from build123d import *

# Parameters (mm, degrees)
CUT_EXTRUDE1_DEPTH       = 12.7
SKETCH10_W               = 4.827435186
SKETCH10_H               = 6.985
FILLET1_R                = 5.08
CIRPATTERN1_COUNT        = 6
FILLET1_OF_CIRPATTERN1_R = 5.08
FILLET2_R                = 0.762
FILLET3_R                = 0.508


with BuildPart() as part:
    # Sketch1 → Revolve1 (revolve)
    with BuildSketch(Plane.XY, mode=Mode.PRIVATE) as revolve1_sk:
        Polygon((71.12, 36.5125), (71.12, 15.5575), (75.565, 15.5575), (75.565, 6.0325), (64.77, 6.0325), (64.77, 18.7325), (67.818, 18.7325), (67.818, 21.9075), (64.77, 21.9075), (64.77, 36.5125), align=None)
    revolve(revolve1_sk.sketch.rotate(Axis((0, 60.757954545, 0), (0, -1, 0)), 180), axis=Axis((0, 60.757954545, 0), (0, -1, 0)))

    # Sketch2 → Cut-Extrude1 (cut)
    with BuildSketch(Plane(origin=(0, 36.5125, 0), x_dir=(1, 0, 0), z_dir=(0, 1, 0))):
        with BuildLine():
            Line((-8.659215821, -70.590880299), (-8.659215821, -65.726040634))
            ThreePointArc((-8.659215821, -65.726040634), (-5.173944735, -66.0917902), (-1.674215821, -66.272855962))
            Line((-1.674215821, -66.272855962), (-1.674215821, -71.100291148))
            ThreePointArc((-1.674215821, -71.100291148), (-5.172990163, -70.931618992), (-8.659215821, -70.590880299))
        make_face()
    cut_extrude1 = extrude(amount=-CUT_EXTRUDE1_DEPTH, mode=Mode.SUBTRACT)

    # Cut-Sweep2: sweep along a path in Sketch23
    with BuildLine(Plane(origin=(0, 23.8125, 0), x_dir=(1, 0, 0), z_dir=(0, 1, 0))) as cut_sweep2_path:
        ThreePointArc((-1.674215821, -71.100291148), (11.313422518, -70.214392192), (23.922019276, -66.976050897))
    # Sketch10 → Cut-Sweep2 (sweep, cut)
    with BuildSketch(Plane.ZY.offset(1.674215821)):
        with Locations((68.686573555, 27.305)):
            Rectangle(SKETCH10_W, SKETCH10_H)
    cut_sweep2 = sweep(path=cut_sweep2_path.line, mode=Mode.SUBTRACT)

    # Fillet1
    fillet1_edges = [part.edges().sort_by_distance(p)[0] for p in [
        (-1.674215821, 30.7975, 68.686573555),
    ]]
    fillet(fillet1_edges, radius=FILLET1_R)

    # CirPattern1: Cut-Extrude1, Cut-Sweep2 ×6 about axis
    cirpattern1_axis = Axis((0, 0, 0), (0, 1, 0))
    add([cut_extrude1.rotate(cirpattern1_axis, i * 360 / CIRPATTERN1_COUNT) for i in range(1, CIRPATTERN1_COUNT)], mode=Mode.SUBTRACT)
    add([cut_sweep2.rotate(cirpattern1_axis, i * 360 / CIRPATTERN1_COUNT) for i in range(1, CIRPATTERN1_COUNT)], mode=Mode.SUBTRACT)

    # Fillet1 of CirPattern1
    fillet1_of_cirpattern1_edges = [part.edges().sort_by_distance(p)[0] for p in [
        (58.647209687, 30.7975, 35.79320021),
        (60.321425508, 30.7975, -32.893373346),
        (1.674215821, 30.7975, -68.686573555),
        (-58.647209687, 30.7975, -35.79320021),
        (-60.321425508, 30.7975, 32.893373346),
    ]]
    fillet(fillet1_of_cirpattern1_edges, radius=FILLET1_OF_CIRPATTERN1_R)

    # Fillet2
    fillet2_edges = [part.edges().sort_by_distance(p)[0] for p in [
        (67.818, 21.9075, 0),
        (67.818, 18.7325, 0),
    ]]
    fillet(fillet2_edges, radius=FILLET2_R)

    # Fillet3
    fillet3_edges = [part.edges().sort_by_distance(p)[0] for p in [
        (64.77, 21.9075, 0),
        (64.77, 18.7325, 0),
    ]]
    fillet(fillet3_edges, radius=FILLET3_R)


solid = part.part
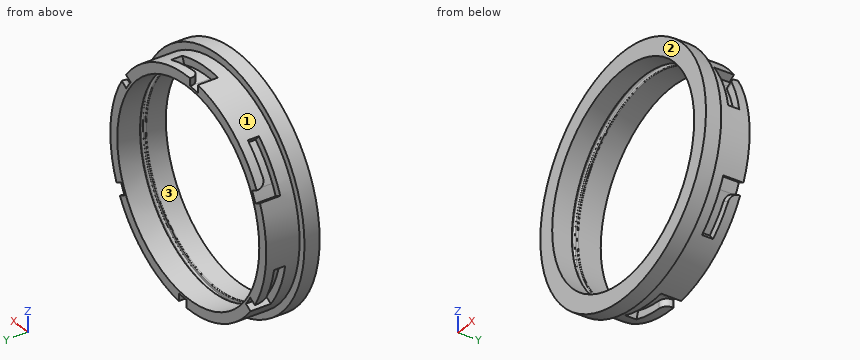
Check sheet for the modelled part. Datum: model origin and axes. Units: mm. Face numbers are marked on the shaded views. Coordinates: 2 decimals unless noted, no trailing zeros. Loops run counter-clockwise (first coordinate to the right, second up) from the corner with the lowest first, then second, coordinate; pieces in that order, holes last. Notation, with made-up numbers: (-26, 57) -> (-15, 57) arc R15 cw to (-15, 73) -> close; hole circle Ø2 at (-35, 33). An arc over 180 degrees is marked (long way). Answer in a Markdown table with one row per item.
1. Release check for a two-part mould opening along X. For the marked faces 1, 2 and 3 record: released by +X, released by -X, zero draft, split by the parting line, or undercut.
Check values:
| item | result |
|---|---|
| face 1 | split by the parting line |
| face 2 | zero draft |
| face 3 | undercut |
2. Sectioned sample at B-B, the plane y = 10.5. Record the boundary of the cut face in (x, z) (3 decimals), then the cut area to 3 significant figures.
Check values:
| item | result |
|---|---|
| outline | circle Ø151.13 at (0, 0); hole circle Ø129.54 at (0, 0) |
| area | 4,760 mm2 |
3. Go/stop test with flat-tipped pins: pin 1 (12 mm diameter, centred on y = 19.5, z = -4, fed in from +X) (3 decimals); pin 2 (1.5 mm diameter, centred on x = 58, y = 10, fed in from +Z); pin 3 (4 mm diameter, centred on y = 18.5, z = -53.5, fed in from -X); pin 4 (5.5 mm diameter, centred on y = 30, z = -68, fed in from -X). Record where each tip stops, or that it passes through.
Check values:
| item | result |
|---|---|
| pin 1 | stops at x = 75.565 |
| pin 2 | stops at z = 49.32 |
| pin 3 | stops at x = -49.05 |
| pin 4 | stops at x = -28.29 |
4. Sectioned sample at A-A, the plane z = 0. Record the boundary of the cut face in (x, y) (1 decimal).
Check values:
| item | result |
|---|---|
| outline | (-75.6, 6) -> (-64.8, 6) -> (-64.8, 18.2) arc R0.5 ccw to (-65.3, 18.7) -> (-67.1, 18.7) arc R0.8 cw to (-67.8, 19.5) -> (-67.8, 21.1) arc R0.8 cw to (-67.1, 21.9) -> (-65.3, 21.9) arc R0.5 ccw to (-64.8, 22.4) -> (-64.8, 36.5) -> (-71.1, 36.5) -> (-71.1, 15.6) -> (-75.6, 15.6) -> close; (64.8, 6) -> (75.6, 6) -> (75.6, 15.6) -> (71.1, 15.6) -> (71.1, 36.5) -> (64.8, 36.5) -> (64.8, 22.4) arc R0.5 ccw to (65.3, 21.9) -> (67.1, 21.9) arc R0.8 cw to (67.8, 21.1) -> (67.8, 19.5) arc R0.8 cw to (67.1, 18.7) -> (65.3, 18.7) arc R0.5 ccw to (64.8, 18.2) -> close |
5. Material ranges on line 1 along Z through (x, y) = (0, 20.1); line 2 along Z through (x, y) = (0, 14.75) (3 decimals); line 3 along X through (y, z) = (9.5, -44), recorded low to high. Write a range as [from, to].
Check values:
| item | result |
|---|---|
| line 1 | z = [-71.12, -67.82], [67.82, 71.12] |
| line 2 | z = [-75.565, -64.77], [64.77, 75.565] |
| line 3 | x = [-61.43, -47.53], [47.53, 61.43] |
